```python
from build123d import *

# Parameters (mm, degrees)
EXTRUDE_1_DEPTH            = 26
CUT_EXTRUDE_1_DEPTH        = 23
CUT_EXTRUDE_2_DEPTH        = 1.6
EXTRUDE_START              = 5.5
EXTRUDE_2_DEPTH            = 5.5
EXTRUDE_START_2            = 17.5
EXTRUDE_3_DEPTH            = 8
CUT_EXTRUDE_3_DEPTH        = 1.6
SKETCH_10_W                = 10
SKETCH_10_H                = 5
EXTRUDE_4_DEPTH            = 5
SKETCH_11_R                = 1.5
CUT_EXTRUDE_4_DEPTH        = 70.108610173
CHAMFER_1_SIZE             = 1.5
CHAMFER_1_OF_MIRROR_2_SIZE = 1.5
MIRROR_START               = -25
MIRROR_3_OUTLINE_R         = 1.5
MIRROR_3_DEPTH             = 5
CUT_EXTRUDE1_START         = 1.5
CUT_EXTRUDE1_DEPTH         = 5
CUT_EXTRUDE_5_DEPTH        = 0.7
CUT_EXTRUDE_6_DEPTH        = 1
SKETCH_16_W                = 13
SKETCH_16_H                = 9.5
CUT_EXTRUDE_10_DEPTH       = 0.5


# Read off the part's stored shape, not the designer's step: Зеркальное отражение3
with BuildPart() as part:
    # Эскиз1 → Бобышка-Вытянуть1 (new body)
    with BuildSketch(Plane.XY):
        with BuildLine():
            Line((-38, -25), (38, -25))
            ThreePointArc((38, -25), (39.414213562, -24.414213562), (40, -23))
            Line((40, -23), (40, 23))
            ThreePointArc((40, 23), (39.414213562, 24.414213562), (38, 25))
            Line((38, 25), (-38, 25))
            ThreePointArc((-38, 25), (-39.414213562, 24.414213562), (-40, 23))
            Line((-40, 23), (-40, -23))
            ThreePointArc((-40, -23), (-39.414213562, -24.414213562), (-38, -25))
        make_face()
    extrude(amount=EXTRUDE_1_DEPTH)

    # Эскиз4 → Вырез-Вытянуть1 (cut)
    with BuildSketch(Plane.XY.offset(26)):
        with BuildLine():
            Line((-33, 22), (33, 22))
            ThreePointArc((33, 22), (35.956795679, 19.507305936), (34, 16.171572875))
            Line((34, 16.171572875), (34, 13.509108241))
            Line((34, 13.509108241), (34, -18))
            ThreePointArc((34, -18), (32.828427125, -20.828427125), (30, -22))
            Line((30, -22), (-30, -22))
            ThreePointArc((-30, -22), (-32.828427125, -20.828427125), (-34, -18))
            Line((-34, -18), (-34, 13.509108241))
            Line((-34, 13.509108241), (-34, 16.171572875))
            ThreePointArc((-34, 16.171572875), (-35.956795679, 19.507305936), (-33, 22))
        make_face()
    extrude(amount=-CUT_EXTRUDE_1_DEPTH, mode=Mode.SUBTRACT)

    # Эскиз6 → Вырез-Вытянуть2 (cut)
    with BuildSketch(Plane.XY.offset(26)):
        with BuildLine():
            Line((-36.5, 23.5), (36.5, 23.5))
            ThreePointArc((36.5, 23.5), (37.914213562, 22.914213562), (38.5, 21.5))
            Line((38.5, 21.5), (38.5, -21.5))
            ThreePointArc((38.5, -21.5), (37.914213562, -22.914213562), (36.5, -23.5))
            Line((36.5, -23.5), (-36.5, -23.5))
            ThreePointArc((-36.5, -23.5), (-37.914213562, -22.914213562), (-38.5, -21.5))
            Line((-38.5, -21.5), (-38.5, 21.5))
            ThreePointArc((-38.5, 21.5), (-37.914213562, 22.914213562), (-36.5, 23.5))
        make_face()
    extrude(amount=-CUT_EXTRUDE_2_DEPTH, mode=Mode.SUBTRACT)

    # Эскиз7 → Бобышка-Вытянуть2 (add)
    with BuildSketch(Plane.XY.offset(3).offset(EXTRUDE_START)):
        with BuildLine():
            Line((-27.5, -6), (-30, -6))
            ThreePointArc((-30, -6), (-32.828427125, -4.828427125), (-34, -2))
            Line((-34, -2), (-34, -18))
            ThreePointArc((-34, -18), (-32.828427125, -20.828427125), (-30, -22))
            Line((-30, -22), (-27.5, -22))
            ThreePointArc((-27.5, -22), (-31.5, -18), (-27.5, -14))
            Line((-27.5, -14), (-27.5, -6))
        make_face()
    extrude_2 = extrude(amount=-EXTRUDE_2_DEPTH)

    # Зеркальное отражение4: Бобышка-Вытянуть2 across plane
    add(extrude_2.mirror(Plane(origin=(0, 0, 0), x_dir=(0, 0, 1), z_dir=(1, 0, 0))))

    # Эскиз8 → Бобышка-Вытянуть3 (add)
    with BuildSketch(Plane(origin=(0, 0, 0), x_dir=(0, 0, -1), z_dir=(1, 0, 0)).offset(EXTRUDE_START_2)):
        Polygon((-6, 7.136038969), (-3, 7.136038969), (-3, 4.136038969), (-7, 4.136038969), (-7, 6.136038969), align=None)
    extrude_3 = extrude(amount=EXTRUDE_3_DEPTH)

    # Зеркальное отражение1: Бобышка-Вытянуть3 across plane
    add(extrude_3.mirror(Plane(origin=(0, 0, 0), x_dir=(0, 0, 1), z_dir=(1, 0, 0))))

    # Эскиз9 → Вырез-Вытянуть3 (cut)
    with BuildSketch(Plane.XY.offset(24.4)):
        with BuildLine():
            Line((-36.5, -23.5), (36.5, -23.5))
            ThreePointArc((36.5, -23.5), (37.914213562, -22.914213562), (38.5, -21.5))
            Line((38.5, -21.5), (38.5, -1))
            ThreePointArc((38.5, -1), (37.914213562, 0.414213562), (36.5, 1))
            Line((36.5, 1), (-36.5, 1))
            ThreePointArc((-36.5, 1), (-37.914213562, 0.414213562), (-38.5, -1))
            Line((-38.5, -1), (-38.5, -21.5))
            ThreePointArc((-38.5, -21.5), (-37.914213562, -22.914213562), (-36.5, -23.5))
        make_face()
    extrude(amount=-CUT_EXTRUDE_3_DEPTH, mode=Mode.SUBTRACT)

    # Эскиз10 → Бобышка-Вытянуть4 (add)
    with BuildSketch(Plane(origin=(0, 0, 0), x_dir=(-1, 0, 0), z_dir=(0, 0, -1))):
        with Locations((-27.5, 22.5)):
            Rectangle(SKETCH_10_W, SKETCH_10_H)
    extrude_4 = extrude(amount=EXTRUDE_4_DEPTH)

    # Эскиз11 → Вырез-Вытянуть4 (cut, through all)
    with BuildSketch(Plane(origin=(0, 25, 0), x_dir=(1, 0, 0), z_dir=(0, 1, 0))):
        with Locations(Location((27.5, 1.6, 0), (0, 0, 180))):
            Circle(SKETCH_11_R)
    cut_extrude_4 = extrude(amount=-CUT_EXTRUDE_4_DEPTH, mode=Mode.SUBTRACT)

    # Фаска1
    chamfer_1_edges = [part.edges().sort_by_distance(p)[0] for p in [
        (32.5, 22.5, -5),
        (22.5, 22.5, -5),
    ]]
    chamfer(chamfer_1_edges, length=CHAMFER_1_SIZE)

    # Зеркальное отражение2: Бобышка-Вытянуть4, Вырез-Вытянуть4 across plane
    add(extrude_4.mirror(Plane(origin=(0, 0, 0), x_dir=(0, 0, 1), z_dir=(1, 0, 0))))
    add(cut_extrude_4.mirror(Plane(origin=(0, 0, 0), x_dir=(0, 0, 1), z_dir=(1, 0, 0))), mode=Mode.SUBTRACT)

    # Фаска1 of Зеркальное отражение2
    chamfer_1_of_mirror_2_edges = [part.edges().sort_by_distance(p)[0] for p in [
        (-32.5, 22.5, -5),
        (-22.5, 22.5, -5),
    ]]
    chamfer(chamfer_1_of_mirror_2_edges, length=CHAMFER_1_OF_MIRROR_2_SIZE)

    # Зеркальное отражение3 outline → Зеркальное отражение3 (add)
    # profile 1 of 2: a face of its own
    with BuildSketch(Plane(origin=(0, 0, 0), x_dir=(1, 0, 0), z_dir=(0, 1, 0)).offset(MIRROR_START)):
        Polygon((22.5, 0), (32.5, 0), (32.5, 3.5), (31, 5), (24, 5), (22.5, 3.5), align=None)
        with Locations((27.5, 1.6)):
            Circle(MIRROR_3_OUTLINE_R, mode=Mode.SUBTRACT)
    # profile 2 of 2: a face of its own
    with BuildSketch(Plane(origin=(0, 0, 0), x_dir=(1, 0, 0), z_dir=(0, 1, 0)).offset(MIRROR_START)):
        Polygon((-32.5, 0), (-22.5, 0), (-22.5, 3.5), (-24, 5), (-31, 5), (-32.5, 3.5), align=None)
        with Locations((-27.5, 1.6)):
            Circle(MIRROR_3_OUTLINE_R, mode=Mode.SUBTRACT)
    extrude(amount=MIRROR_3_DEPTH)

    # Sketch1 → Cut-Extrude1 (cut)
    with BuildSketch(Plane.XY.offset(8.5).offset(CUT_EXTRUDE1_START)):
        with BuildLine():
            Line((35, 12), (35, -6))
            ThreePointArc((35, -6), (34.746427842, -8.121320344), (34, -10.123105626))
            Line((34, -10.123105626), (34, 16.123105626))
            ThreePointArc((34, 16.123105626), (34.746427842, 14.121320344), (35, 12))
        make_face()
    cut_extrude1 = extrude(amount=CUT_EXTRUDE1_DEPTH, mode=Mode.SUBTRACT)

    # Mirror1: Cut-Extrude1 across plane
    add(cut_extrude1.mirror(Plane(origin=(0, 0, 0), x_dir=(0, 0, 1), z_dir=(1, 0, 0))), mode=Mode.SUBTRACT)

    # Эскиз13 → Вырез-Вытянуть5 (cut)
    with BuildSketch(Plane.XY.offset(3)):
        with BuildLine():
            Line((15.5, 4), (16.5, 4))
            ThreePointArc((16.5, 4), (19.328427125, 2.828427125), (20.5, 0))
            Line((20.5, 0), (20.5, -17))
            ThreePointArc((20.5, -17), (19.328427125, -19.828427125), (16.5, -21))
            Line((16.5, -21), (1.5, -21))
            ThreePointArc((1.5, -21), (-1.328427125, -19.828427125), (-2.5, -17))
            Line((-2.5, -17), (-2.5, 0))
            ThreePointArc((-2.5, 0), (-1.328427125, 2.828427125), (1.5, 4))
            Line((1.5, 4), (2.5, 4))
            Line((2.5, 4), (15.5, 4))
        make_face()
    extrude(amount=-CUT_EXTRUDE_5_DEPTH, mode=Mode.SUBTRACT)

    # Эскиз14 → Вырез-Вытянуть6 (cut)
    with BuildSketch(Plane.XY.offset(3)):
        with BuildLine():
            Line((-30, 22), (20, 22))
            ThreePointArc((20, 22), (24.25, 17.75), (20, 13.5))
            Line((20, 13.5), (-30, 13.5))
            ThreePointArc((-30, 13.5), (-34.25, 17.75), (-30, 22))
        make_face()
    extrude(amount=-CUT_EXTRUDE_6_DEPTH, mode=Mode.SUBTRACT)

    # Эскиз16 → Вырез-Вытянуть10 (cut)
    with BuildSketch(Plane.XY.offset(3)):
        with Locations((9, 8.75)):
            Rectangle(SKETCH_16_W, SKETCH_16_H)
    extrude(amount=-CUT_EXTRUDE_10_DEPTH, mode=Mode.SUBTRACT)


solid = part.part
```
Could you check a few things on this model? Use its own coordinates, in mm. A direction names the side the tool comes from. Round coordinates to 2 decimals unless told otherwise and drop trailing zeros. Loops run counter-clockwise (first coordinate to the right, second up) from the corner with the lowest first, then second, coordinate; pieces in that order, holes last. Notation, with made-up numbers: M 17,4.25 L 60,4.25 A14 cw 60,31.25 Z; hole C 24.25,66 d1. An arc over 180 degrees is marked long. Write item = value, one per line.
1. I want a section at A-A, the plane z = 11. Write out the boundary of the cut face in (x, y).
Results below:
outline = M -40,-23 A2 ccw -38,-25 L 38,-25 A2 ccw 40,-23 L 40,23 A2 ccw 38,25 L -38,25 A2 ccw -40,23 Z; hole M -35,-6 A9 ccw -34,-10.12 L -34,-18 A4 ccw -30,-22 L 30,-22 A4 ccw 34,-18 L 34,-10.12 A9 ccw 35,-6 L 35,12 A9 ccw 34,16.12 L 34,16.17 A3 ccw 33,22 L -33,22 A3 ccw -34,16.17 L -34,16.12 A9 ccw -35,12 Z
2. I want a section at D-D, the plane y = 17.75. Write out the boundary of the cut face in (x, z).
Results below:
outline = M -40,0 L 40,0 L 40,26 L 38.5,26 L 38.5,24.4 L 35.73,24.4 L 35.73,3 L 24.25,3 L 24.25,2 L -34.25,2 L -34.25,3 L -35.73,3 L -35.73,24.4 L -38.5,24.4 L -38.5,26 L -40,26 Z
3. Thinking about a two-plate mould opening in Y: for faces 4 (the face through (-28, 20, -4)), 5 (the face through (-32.5, -23, -2)), which applies, +Y half, -Y half, draft (parallel to the pull), parting line (faces both ways), or undercut?
Results below:
face_4 = undercut
face_5 = draft
4. Which directions (+Z, -Z, +X, -X, +Y, -Y) give clear straight access to the entire face, cutting with the end or side of a thin tool? Please do faces 1 (the face through (23, 22, -4)), 2 (the face through (-27, -23, -5)), 3 (the face through (32.797, -4.859, 5.788)).
Results below:
face_1 = -Z, +Y, -Y
face_2 = -Z, +X, -X, +Y, -Y
face_3 = +Z
5. I want a section at B-B, the plane z = -1.6. Count the separate pieces of the cut face and the enclosed holes in it, and give its area (3 significant figures).
Results below:
separate_pieces = 8
enclosed_holes = 0
area = 140 mm²
6. I want a section at C-C, the plane x = -21.5. Write out the boundary of the cut face in (y, z).
Results below:
outline = M -25,0 L 25,0 L 25,26 L 23.5,26 L 23.5,24.4 L 22,24.4 L 22,2 L 13.5,2 L 13.5,3 L 7.14,3 L 7.14,6 L 6.14,7 L 4.14,7 L 4.14,3 L -22,3 L -22,22.8 L -23.5,22.8 L -23.5,26 L -25,26 Z
7. I need wall thicknesses on probe 1 along X at (y, z) = (-22.3, -1.6); probe 2 along Y at (x, z) = (18, 17); probe 3 along X at (y, z) = (12, 11.5). Which ranges of each line are inside material? Lowest first, please.
Results below:
probe_1 = -32.5 to -29, -26 to -22.5, 22.5 to 26, 29 to 32.5
probe_2 = -25 to -22, 22 to 25
probe_3 = -40 to -35, 35 to 40
8. Will these pins go through, and if not, where does the flat tip stop? P1, Ø19.5, axis at x = 11.5, y = 12, coming from the +Z side; P2, Ø4, axis at y = -22, z = -1, coming from the +X side; P3, Ø15, axis at x = 9.5, y = 6, coming from the -Z side; P4, Ø1.5, axis at x = -31, y = 2.5, coming from the +Z side.
Results below:
P1 = 7
P2 = 40
P3 = 0
P4 = 3
